Read the model definition and answer for the solid it produces. Units are mm, in the model's axes. Face numbers are marked on the shaded views. A direction names the side the tool comes from. Coordinates: 2 decimals unless noted, no trailing zeros. Order: outer loops, then holes, each group sorted by start corner. A loop starts at its lowest first (then second) coordinate and runs counter-clockwise, first axis right, second up. Notation, with made-up numbers: M 88.5,84 L 104.5,84 A10 cw 104.5,103 Z; hole C 3,41.25 d11. An arc over 180 degrees is marked long. Write each question's results on one line, items separated by ' | '.
```python
from build123d import *

# Parameters (mm, degrees)
SKETCH1_W           = 65
SKETCH1_H           = 115
SKETCH1_W_2         = 55
SKETCH1_H_2         = 105
BOSS_EXTRUDE1_DEPTH = 23
FILLET1_R           = 6
SKETCH2_R           = 6
BOSS_EXTRUDE2_DEPTH = 23
SKETCH4_R           = 2.2
CUT_EXTRUDE1_DEPTH  = 23


with BuildPart() as part:
    # Sketch1 → Boss-Extrude1 (new body)
    with BuildSketch(Plane(origin=(0, 0, 0), x_dir=(1, 0, 0), z_dir=(0, 1, 0))):
        Rectangle(SKETCH1_W, SKETCH1_H)
        Rectangle(SKETCH1_W_2, SKETCH1_H_2, mode=Mode.SUBTRACT)
    extrude(amount=BOSS_EXTRUDE1_DEPTH)

    # Fillet1
    fillet1_edges = [part.edges().sort_by_distance(p)[0] for p in [
        (32.5, 11.5, 57.5),
        (-32.5, 11.5, 57.5),
        (-32.5, 11.5, -57.5),
        (32.5, 11.5, -57.5),
    ]]
    fillet(fillet1_edges, radius=FILLET1_R)

    # Sketch2 → Boss-Extrude2 (add)
    with BuildSketch(Plane(origin=(0, 23, 0), x_dir=(1, 0, 0), z_dir=(0, 1, 0))):
        with Locations((-26.5, 51.5)):
            Circle(SKETCH2_R)
        with Locations((26.5, 51.5)):
            Circle(SKETCH2_R)
        with Locations((-26.5, -51.5)):
            Circle(SKETCH2_R)
        with Locations((26.5, -51.5)):
            Circle(SKETCH2_R)
    extrude(amount=-BOSS_EXTRUDE2_DEPTH)

    # Sketch4 → Cut-Extrude1 (cut)
    with BuildSketch(Plane(origin=(0, 23, 0), x_dir=(1, 0, 0), z_dir=(0, 1, 0))):
        with Locations(Location((-26.5, 51.5, 0), (0, 0, 270))):
            Circle(SKETCH4_R)
        with Locations(Location((26.5, 51.5, 0), (0, 0, 270))):
            Circle(SKETCH4_R)
        with Locations(Location((26.5, -51.5, 0), (0, 0, 270))):
            Circle(SKETCH4_R)
        with Locations(Location((-26.5, -51.5, 0), (0, 0, 270))):
            Circle(SKETCH4_R)
    extrude(amount=-CUT_EXTRUDE1_DEPTH, mode=Mode.SUBTRACT)


solid = part.part
```
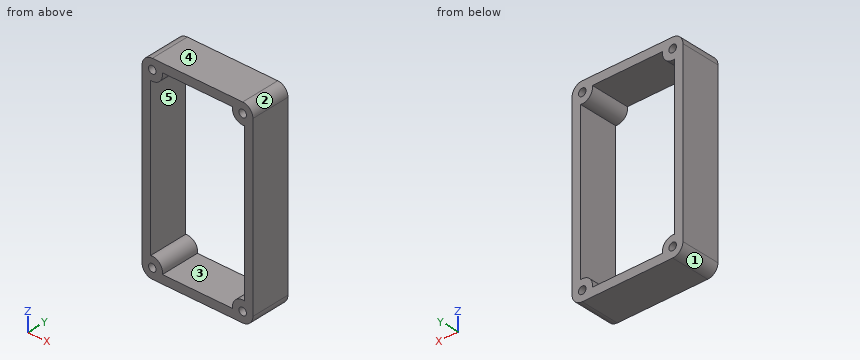
(1) The part is cut by section A-A, the plane z = 6. Write down the section's boundary in (x, y).
Conclusion:
outline: M -32.5,0 L -27.5,0 L -27.5,23 L -32.5,23 Z; M 27.5,0 L 32.5,0 L 32.5,23 L 27.5,23 Z
(2) For the marked faces 4 and 5, determine the directions among +Z, -Z, +X, -X, +Y, -Y from which every point of the face is accessible in a straight line to the end or side of a thin tool.
Conclusion:
face 4: +Z, +X, -X, +Y, -Y | face 5: +Y, -Y
(3) The mould has two halves that part along Z. Classify the marked faces 1, 2 and 3: pulls with the +Z half, pulls with the -Z half, needs draft (parallel to the pull), parting line crosses it, or undercut.
Conclusion:
face 1: pulls with the -Z half | face 2: pulls with the +Z half | face 3: undercut
(4) Straight lines are drawn through the part: line 1 (X direction, y = 13, z = -51.5); line 2 (X direction, y = 2.25, z = -24.5); line 3 (Z direction, x = 4.5, y = 3.75). For each, find the intervals that lie inside material, in ascending order.
Conclusion:
line 1: -32.5 to -28.7, -24.3 to -20.5, 20.5 to 24.3, 28.7 to 32.5 | line 2: -32.5 to -27.5, 27.5 to 32.5 | line 3: -57.5 to -52.5, 52.5 to 57.5
(5) The part is cut by section B-B, the plane x = -4.5. Write down the section's boundary in (y, z), then the cut area to 3 significant figures.
Conclusion:
outline: M 0,-57.5 L 23,-57.5 L 23,-52.5 L 0,-52.5 Z; M 0,52.5 L 23,52.5 L 23,57.5 L 0,57.5 Z | area: 230 mm²
(6) The part is cut by section C-C, the plane y = 2.75. Write down the section's boundary in (x, z), then the cut area to 3 significant figures.
Conclusion:
outline: M -32.5,-51.5 A6 ccw -26.5,-57.5 L 26.5,-57.5 A6 ccw 32.5,-51.5 L 32.5,51.5 A6 ccw 26.5,57.5 L -26.5,57.5 A6 ccw -32.5,51.5 Z; hole C -26.5,-51.5 d4.4; hole C -26.5,51.5 d4.4; hole M -27.5,-45.58 A6 cw -20.58,-52.5 L 20.58,-52.5 A6 cw 27.5,-45.58 L 27.5,45.58 A6 cw 20.58,52.5 L -20.58,52.5 A6 cw -27.5,45.58 Z; hole C 26.5,-51.5 d4.4; hole C 26.5,51.5 d4.4 | area: 1,770 mm²
